Source: CAD feature listing. Evaluate the final solid. Frame: model axes, mm. Give positions to 0.01 mm unless a question says otherwise; leave off trailing zeros. Write each loop counter-clockwise with the first axis right and the second up, starting at its lowest first coordinate (ties: lowest second). Pieces come first, ordered by that corner, then holes. Notation, with made-up numbers: M -15.75,27 L 18.25,27 A26 cw 18.25,50 Z; hole C 41,73 d9. An arc over 180 degrees is marked long. Answer as a JSON object with one key per item and string values. Group by question number.
```python
from build123d import *

# Parameters (mm, degrees)
F1_DEPTH = 1.5


with BuildPart() as f1:
    # F0 (on Top) → F1 (new body)
    with BuildSketch(Plane.XY):
        with BuildLine():
            ThreePointArc((-11.0335932724, 0), (-9.5, 1.5335932724), (-7.9664067276, 0))
            Line((-7.9664067276, 0), (-4.6, 0))
            ThreePointArc((-4.6, 0), (-3.2526911935, 3.2526911935), (0, 4.6))
            Line((0, 4.6), (0, 7.9664067276))
            ThreePointArc((0, 7.9664067276), (-1.5335932724, 9.5), (0, 11.0335932724))
            Line((0, 11.0335932724), (0, 12.2052515495))
            ThreePointArc((0, 12.2052515495), (-0.4345010394, 12.1317339839), (-0.8145803081, 11.9087188829))
            ThreePointArc((-0.8145803081, 11.9087188829), (-0.9635912872, 11.7146325201), (-1.1134019503, 11.5211627464))
            ThreePointArc((-1.1134019503, 11.5211627464), (-6.0214332546, 5.9647454006), (-11.5844815273, 1.064231252))
            ThreePointArc((-11.5844815273, 1.064231252), (-11.7185491453, 0.9605716693), (-11.8529124882, 0.8572956927))
            ThreePointArc((-11.8529124882, 0.8572956927), (-12.1114910997, 0.4629412091), (-12.2012897293, 0))
            Line((-12.2012897293, 0), (-11.0335932724, 0))
        make_face()
        with BuildLine():
            Line((-4.6, 0), (-7.9664067276, 0))
            ThreePointArc((-7.9664067276, 0), (-9.5, -1.5335932724), (-11.0335932724, 0))
            Line((-11.0335932724, 0), (-12.2012897293, 0))
            ThreePointArc((-12.2012897293, 0), (-12.1017179659, -0.4794729938), (-11.8217098669, -0.8812245989))
            ThreePointArc((-11.8217098669, -0.8812245989), (-11.721781237, -0.9580802015), (-11.6220162383, -1.0351480919))
            ThreePointArc((-11.6220162383, -1.0351480919), (-6.0202525949, -5.9659244981), (-1.0822216309, -11.5612941984))
            ThreePointArc((-1.0822216309, -11.5612941984), (-0.9646757294, -11.7132260984), (-0.8476226636, -11.8655380184))
            ThreePointArc((-0.8476226636, -11.8655380184), (-0.4559625925, -12.1137220892), (0, -12.1979305118))
            Line((0, -12.1979305118), (0, -11.0335932724))
            ThreePointArc((0, -11.0335932724), (-1.5335932724, -9.5), (0, -7.9664067276))
            Line((0, -7.9664067276), (0, -4.6))
            ThreePointArc((0, -4.6), (-3.2526911935, -3.2526911935), (-4.6, 0))
        make_face()
        with BuildLine():
            Line((0, 7.9664067276), (0, 4.6))
            ThreePointArc((0, 4.6), (3.2526911935, 3.2526911935), (4.6, 0))
            Line((4.6, 0), (7.9664067276, 0))
            ThreePointArc((7.9664067276, 0), (9.5, 1.5335932724), (11.0335932724, 0))
            Line((11.0335932724, 0), (12.0049398392, 0))
            ThreePointArc((12.0049398392, 0), (11.9193137164, 0.4573515512), (11.6687643937, 0.849432297))
            ThreePointArc((11.6687643937, 0.849432297), (11.5305346329, 0.9577272788), (11.3926261985, 1.0664311591))
            ThreePointArc((11.3926261985, 1.0664311591), (5.8870136821, 6.0076850195), (1.0395559509, 11.5960579882))
            ThreePointArc((1.0395559509, 11.5960579882), (0.9473724033, 11.7171151321), (0.8554998188, 11.838408441))
            ThreePointArc((0.8554998188, 11.838408441), (0.4640913385, 12.1065803567), (0, 12.2052515495))
            Line((0, 12.2052515495), (0, 11.0335932724))
            ThreePointArc((0, 11.0335932724), (1.0844142025, 10.5844142025), (1.5335932724, 9.5))
            ThreePointArc((1.5335932724, 9.5), (1.0844142025, 8.4155857975), (0, 7.9664067276))
        make_face()
        with BuildLine():
            ThreePointArc((4.6, 0), (3.2526911935, -3.2526911935), (0, -4.6))
            Line((0, -4.6), (0, -7.9664067276))
            ThreePointArc((0, -7.9664067276), (1.0844142025, -8.4155857975), (1.5335932724, -9.5))
            ThreePointArc((1.5335932724, -9.5), (1.0844142025, -10.5844142025), (0, -11.0335932724))
            Line((0, -11.0335932724), (0, -12.1979305118))
            ThreePointArc((0, -12.1979305118), (0.4647348704, -12.1017306528), (0.8576533678, -11.8355578385))
            ThreePointArc((0.8576533678, -11.8355578385), (0.9532380505, -11.7093930262), (1.0491591917, -11.5834838282))
            ThreePointArc((1.0491591917, -11.5834838282), (5.9633685423, -5.9301704288), (11.5511297333, -0.9415502985))
            ThreePointArc((11.5511297333, -0.9415502985), (11.8839118623, -0.5218059727), (12.0049398392, 0))
            Line((12.0049398392, 0), (11.0335932724, 0))
            ThreePointArc((11.0335932724, 0), (9.5, -1.5335932724), (7.9664067276, 0))
            Line((7.9664067276, 0), (4.6, 0))
        make_face()
        with BuildLine():
            ThreePointArc((-11.5844815273, 1.064231252), (-11.7259145151, 0.970125819), (-11.8529124882, 0.8572956927))
            ThreePointArc((-11.8529124882, 0.8572956927), (-11.7185491453, 0.9605716693), (-11.5844815273, 1.064231252))
        make_face()
        with BuildLine():
            ThreePointArc((-11.6220162383, -1.0351480919), (-11.721781237, -0.9580802015), (-11.8217098669, -0.8812245989))
            ThreePointArc((-11.8217098669, -0.8812245989), (-11.7258479783, -0.9633562144), (-11.6220162383, -1.0351480919))
        make_face()
        with BuildLine():
            ThreePointArc((-0.8145803081, 11.9087188829), (-0.9836129307, 11.7300700266), (-1.1134019503, 11.5211627464))
            ThreePointArc((-1.1134019503, 11.5211627464), (-0.9635912872, 11.7146325201), (-0.8145803081, 11.9087188829))
        make_face()
        with BuildLine():
            ThreePointArc((-0.8476226636, -11.8655380184), (-0.9646757294, -11.7132260984), (-1.0822216309, -11.5612941984))
            ThreePointArc((-1.0822216309, -11.5612941984), (-0.9769671574, -11.7227038795), (-0.8476226636, -11.8655380184))
        make_face()
        with BuildLine():
            ThreePointArc((1.0395559509, 11.5960579882), (0.9551101208, 11.72299164), (0.8554998188, 11.838408441))
            ThreePointArc((0.8554998188, 11.838408441), (0.9473724033, 11.7171151321), (1.0395559509, 11.5960579882))
        make_face()
        with BuildLine():
            ThreePointArc((1.0491591917, -11.5834838282), (0.9532380505, -11.7093930262), (0.8576533678, -11.8355578385))
            ThreePointArc((0.8576533678, -11.8355578385), (0.9616128176, -11.7157555094), (1.0491591917, -11.5834838282))
        make_face()
        with BuildLine():
            ThreePointArc((11.3926261985, 1.0664311591), (11.5305346329, 0.9577272788), (11.6687643937, 0.849432297))
            ThreePointArc((11.6687643937, 0.849432297), (11.5385404595, 0.9679149567), (11.3926261985, 1.0664311591))
        make_face()
    extrude(amount=F1_DEPTH)


solid = f1.part
```
(1) Contact query for a flat-ended pin moving along its axis: pin 1 Ø1 at (x, y) = (-8, -5.5) entering from +Z. Output: stop coordinate, or through.
(2) Pull-direction query (X, two-part tool) for faces 1 (the cylindrical face through (5.96, 5.934, 0.74)), 2 (the flat face through (-5, 1, 1.5)), 3 (the cylindrical face through (-5.948, 6.038, 0.74)), 4 (the cylindrical face through (-8.037, -0.461, 0.74)); classes: pulls with the +X half, pulls with the -X half, needs draft (parallel to the pull), parting line crosses it, or undercut.
(3) Section B-B, the plane x = -10.25. Return loops of the section in (y, z), plus the area to 3 significant figures.
(4) Section A-A, the plane z = 1.05. Return loops of the section in (x, y), plus the area to 3 significant figures.
(5) Section D-D, the plane x = 6.75. Return loops of the section in (y, z).
(6) Section C-C, the plane y = 9. Return loops of the section in (x, z).
(7) Ray query, L1, parallel to Y at x = 0.5, z = 0.35; L2, parallel to X at y = -8.25, z = 0.3; L3, parallel to Y at x = -9.5, z = 0.6. Return the intervals inside material, ascending. Write a range as [from, to].
Reported:
{
 "1": {"pin 1": "passes through"},
 "2": {"face 1": "pulls with the +X half", "face 2": "needs draft", "face 3": "pulls with the -X half", "face 4": "undercut"},
 "3": {"outline": "M -2.13,0 L -1.34,0 L -1.34,1.5 L -2.13,1.5 Z; M 1.34,0 L 2.13,0 L 2.13,1.5 L 1.34,1.5 Z", "area": "2.38 mm2"},
 "4": {"outline": "M -11.62,-1.04 A59.29 cw -1.08,-11.56 A1.22 ccw 1.05,-11.58 A59.29 cw 11.55,-0.94 A1.22 ccw 11.39,1.07 A59.29 cw 1.04,11.6 A1.22 ccw -1.11,11.52 A59.29 cw -11.58,1.06 A1.22 ccw Z; hole C -9.5,0 d3.07; hole C 0,0 d9.2; hole C 0,-9.5 d3.07; hole C 0,9.5 d3.07; hole C 9.5,0 d3.07", "area": "202 mm2"},
 "5": {"outline": "M -5.15,0 L 5.15,0 L 5.15,1.5 L -5.15,1.5 Z"},
 "6": {"outline": "M -3.19,0 L -1.45,0 L -1.45,1.5 L -3.19,1.5 Z; M 1.45,0 L 3.14,0 L 3.14,1.5 L 1.45,1.5 Z"},
 "7": {"L1": "y = [-12.09, -10.95], [-8.05, -4.57], [4.57, 8.05], [10.95, 12.09]", "L2": "x = [-3.85, -0.89], [0.89, 3.79]", "L3": "y = [-2.76, -1.53], [1.53, 2.76]"}
}
